from build123d import *

# Parameters (mm, degrees)
SKETCH1_W           = 80
SKETCH1_H           = 40
BOSS_EXTRUDE1_DEPTH = 12
SKETCH2_W           = 12
SKETCH2_H           = 40
BOSS_EXTRUDE2_DEPTH = 40
SKETCH3_W           = 40
SKETCH3_H           = 12
BOSS_EXTRUDE3_DEPTH = 40
FILLET1_R           = 20
SKETCH4_R           = 8
CUT_EXTRUDE1_DEPTH  = 12
SKETCH5_R           = 8
CUT_EXTRUDE2_DEPTH  = 12
SKETCH6_R           = 8
CUT_EXTRUDE3_DEPTH  = 80.961215088


with BuildPart() as part:
    # Sketch1 → Boss-Extrude1 (new body)
    with BuildSketch(Plane(origin=(0, 0, 0), x_dir=(1, 0, 0), z_dir=(0, 1, 0))):
        with Locations((5.714285714, -3.314285714)):
            Rectangle(SKETCH1_W, SKETCH1_H)
    extrude(amount=BOSS_EXTRUDE1_DEPTH)

    # Sketch2 → Boss-Extrude2 (add)
    with BuildSketch(Plane(origin=(0, 12, 0), x_dir=(1, 0, 0), z_dir=(0, 1, 0))):
        with Locations((-28.285714286, -3.314285714)):
            Rectangle(SKETCH2_W, SKETCH2_H)
    extrude(amount=BOSS_EXTRUDE2_DEPTH)

    # Sketch3 → Boss-Extrude3 (add)
    with BuildSketch(Plane.XZ):
        with Locations((-14.285714286, 17.314285714)):
            Rectangle(SKETCH3_W, SKETCH3_H)
        with Locations((-14.285714286, -10.685714286)):
            Rectangle(SKETCH3_W, SKETCH3_H)
    extrude(amount=BOSS_EXTRUDE3_DEPTH)

    # Fillet1
    fillet1_edges = [part.edges().sort_by_distance(p)[0] for p in [
        (-34.285714286, -40, -10.685714286),
        (-34.285714286, -40, 17.314285714),
        (5.714285714, -40, -10.685714286),
        (5.714285714, -40, 17.314285714),
        (45.714285714, 6, -16.685714286),
        (45.714285714, 6, 23.314285714),
        (-28.285714286, 52, -16.685714286),
        (-28.285714286, 52, 23.314285714),
    ]]
    fillet(fillet1_edges, radius=FILLET1_R - 0.0001)  # a hair under: the kernel refuses the full size

    # Sketch4 → Cut-Extrude1 (cut)
    with BuildSketch(Plane(origin=(-22.285714286, 0, 0), x_dir=(0, 0, -1), z_dir=(1, 0, 0))):
        with Locations((-3.314285714, 32)):
            Circle(SKETCH4_R)
    extrude(amount=-CUT_EXTRUDE1_DEPTH, mode=Mode.SUBTRACT)

    # Sketch5 → Cut-Extrude2 (cut)
    with BuildSketch(Plane(origin=(0, 12, 0), x_dir=(1, 0, 0), z_dir=(0, 1, 0))):
        with Locations(Location((25.714285714, -3.314285714, 0), (0, 0, 270))):
            Circle(SKETCH5_R)
    extrude(amount=-CUT_EXTRUDE2_DEPTH, mode=Mode.SUBTRACT)

    # Sketch6 → Cut-Extrude3 (cut, through all)
    with BuildSketch(Plane.XY.offset(23.314285714)):
        with Locations((-14.285714286, -20)):
            Circle(SKETCH6_R)
    extrude(amount=-CUT_EXTRUDE3_DEPTH, mode=Mode.SUBTRACT)


solid = part.part
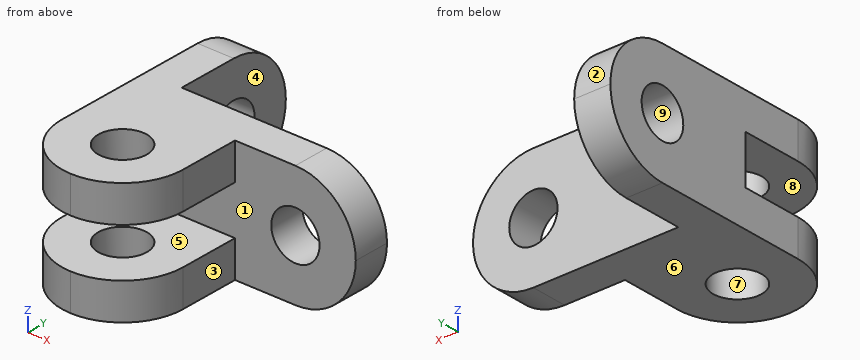
Read the model definition and answer for the solid it produces. Units are mm, in the model's axes. Face numbers are marked on the shaded views. A direction names the side the tool comes from. Round coordinates to 2 decimals unless told otherwise and drop trailing zeros. Order: outer loops, then holes, each group sorted by start corner. A loop starts at its lowest first (then second) coordinate and runs counter-clockwise, first axis right, second up.
1) Flat-ended cylindrical pins translate along their axes: pin 1 (2 mm diameter, centred on y = -20, z = 13.5, fed in from +X); pin 2 (2 mm diameter, centred on y = -22.5, z = -12, fed in from -X); pin 3 (4 mm diameter, centred on x = -15.5, z = -4, fed in from +Y); pin 4 (21 mm diameter, centred on x = -14.29, y = -20, fed in from -Z). Find the tip coordinate at first contact, or state that the pin passes through.
2) The part is cut by section B-B on x = -8.5. Write down the section's boundary in (y, z).
3) For the marked faces 1, 2, 3, 4 and 5, determine the directions among +Z, -Z, +X, -X, +Y, -Y from which every point of the face is accessible in a straight line to the end or side of a thin tool.
4) Straight lines are drawn through the part: L1, parallel to Z at x = -22.5, y = -23; L2, parallel to X at y = 46, z = -2.5; L3, parallel to Y at x = 18, z = -13.5. For each, find the intervals that lie inside material, in ascending order.
5) The mould has two halves that part along Z. Classify the marked faces 6, 7, 8 and 9: released by +Z, released by -Z, zero draft, split by the parting line, or undercut.
6) The part is cut by section A-A on y = -7. Write down the section's boundary in (x, z).
Resolved:
1. pin 1: stops at x = 5.71
1. pin 2: stops at x = -34.23
1. pin 3: stops at y = 12
1. pin 4: stops at z = -16.69
2. outline: (-39.14, -16.69) - (-25.52, -16.69) - (-25.52, -4.69) - (-39.14, -4.69) - close; (-39.14, 11.31) - (-25.52, 11.31) - (-25.52, 23.31) - (-39.14, 23.31) - close; (-14.48, -16.69) - (12, -16.69) - (12, 23.31) - (-14.48, 23.31) - (-14.48, 11.31) - (0, 11.31) - (0, -4.69) - (-14.48, -4.69) - close
3. face 1: +X, -Y
3. face 2: +Z, +X, -X, +Y
3. face 3: +Z, -Z, +X, -Y
3. face 4: +Z, -Z, +X, +Y
3. face 5: +X, -X, -Y
4. L1: z = -16.69 to -4.69, 11.31 to 23.31
4. L2: x = -34.29 to -22.29
4. L3: y = 0 to 12
5. face 6: released by -Z
5. face 7: zero draft
5. face 8: undercut
5. face 9: undercut
6. outline: (-34.29, -16.69) - (5.71, -16.69) - (5.71, -4.69) - (-34.29, -4.69) - close; (-34.29, 11.31) - (5.71, 11.31) - (5.71, 23.31) - (-34.29, 23.31) - close
